```python
from build123d import *

# Parameters (mm, degrees)
STOCK_LED_START                   = -2.54
STOCK_LED_LIGHT_HOUSING_1_DEPTH   = 2.54
STOCK_LED_LIGHT_HOUSING_1_2_DEPTH = 13.97
SKETCH3_W                         = 2.54
SKETCH3_H                         = 17.78
PIECE_UNDER_BATTERY_PLUG_DEPTH    = 7.62
CUT_OUT_FOR_PLUG_REACH            = 94.065
SKETCH4_R                         = 5.157413323
HOLES_FOR_SCREWS_D                = 3.2639
SKETCH7_W                         = 25.4
SKETCH7_H                         = 12.726484406
SKETCH7_W_2                       = 12.813224924
SKETCH7_H_2                       = 12.784135739
NAILS_GO_HERE_DEPTH               = 3.81
NAIL_HOLES_D                      = 3.2639
FILLET1_R                         = 2.54


# Read off the part's stored shape, not the designer's step: Stock-LED Light housing-1
with BuildPart() as part:
    # Stock-LED Light housing-1 outline → Stock-LED Light housing-1 (new body)
    with BuildSketch(Plane(origin=(0, 0, 0), x_dir=(1, 0, 0), z_dir=(0, 1, 0)).offset(STOCK_LED_START)):
        Polygon((71.203772107, -22.802348667), (71.203772107, 38.157651333), (-11.408866572, 38.157651333), (-11.408866572, 0.057651333), (-42.066153873, 0.057651333), (-42.066153873, -22.802348667), align=None)
    extrude(amount=STOCK_LED_LIGHT_HOUSING_1_DEPTH)

    # Stock-LED Light housing-1 2 outline → Stock-LED Light housing-1 2 (add)
    with BuildSketch(Plane(origin=(0, 0, 0), x_dir=(1, 0, 0), z_dir=(0, 1, 0))):
        Polygon((71.203772107, -22.802348667), (71.203772107, 38.157651333), (-11.408866572, 38.157651333), (-11.408866572, 0.057651333), (-42.066153873, 0.057651333), (-42.066153873, -22.802348667), align=None)
        Polygon((-39.526153873, -20.262348667), (-39.526153873, -2.482348667), (-8.868866572, -2.482348667), (-8.868866572, 35.617651333), (68.663772107, 35.617651333), (68.663772107, -20.262348667), align=None, mode=Mode.SUBTRACT)
    extrude(amount=STOCK_LED_LIGHT_HOUSING_1_2_DEPTH)

    # Sketch3 → Piece under battery plug (add)
    with BuildSketch(Plane(origin=(0, 0, 0), x_dir=(1, 0, 0), z_dir=(0, 1, 0))):
        with Locations((-10.138866572, -11.372348667)):
            Rectangle(SKETCH3_W, SKETCH3_H)
    extrude(amount=PIECE_UNDER_BATTERY_PLUG_DEPTH)

    # Sketch4 → Cut out for plug (cut, up to next)
    with BuildSketch(Plane(origin=(-11.408866572, 0, 0), x_dir=(0, 0, -1), z_dir=(1, 0, 0)), mode=Mode.PRIVATE) as cut_out_for_plug_sk1:
        with Locations((-11.372348667, 7.62)):
            Circle(SKETCH4_R)
    cut_out_for_plug_tool1 = extrude(cut_out_for_plug_sk1.sketch, amount=CUT_OUT_FOR_PLUG_REACH, mode=Mode.PRIVATE) & part.part
    add(cut_out_for_plug_tool1.solids().sort_by_distance((-11.408867, 7.62, 11.372349))[0], mode=Mode.SUBTRACT)

    # holes for screws (through all)
    with Locations(Plane(origin=(0, 0, 0), x_dir=(1, 0, 0), z_dir=(0, 1, 0))):
        with Locations((14.053772107, 31.922137324), (12.783772107, -16.337862676), (64.853772107, -11.257862676), (64.853772107, 16.682137324)):
            Hole(HOLES_FOR_SCREWS_D / 2)

    # Sketch7 → Nails go here (add)
    with BuildSketch(Plane(origin=(0, 13.97, 0), x_dir=(1, 0, 0), z_dir=(0, 1, 0))):
        with Locations((-24.108866572, 6.420893536)):
            Rectangle(SKETCH7_W, SKETCH7_H)
        with Locations((77.610384569, 6.39206787)):
            Rectangle(SKETCH7_W_2, SKETCH7_H_2)
    extrude(amount=-NAILS_GO_HERE_DEPTH)

    # Nail holes (through all)
    with Locations(Plane(origin=(0, 10.16, 0), x_dir=(-1, 0, 0), z_dir=(0, -1, 0))):
        with Locations((30.430786564, 6.434135739), (-77.666997031, 6.434135739)):
            Hole(NAIL_HOLES_D / 2)

    # Fillet1
    fillet1_edges = [part.edges().sort_by_distance(p)[0] for p in [
        (71.203772107, 5.715, -38.157651333),
        (71.203772107, 5.715, 22.802348667),
        (-36.808866572, 10.16, -6.420893536),
        (-24.108866572, 10.16, -12.784135739),
        (-36.808866572, 12.065, -12.784135739),
        (77.610384569, 10.16, -12.784135739),
        (84.016997031, 10.16, -6.392067869),
        (84.016997031, 12.065, -12.784135739),
        (77.610384569, 10.16, 0),
        (84.016997031, 12.065, 0),
        (-26.737510222, -2.54, -0.057651333),
        (14.568809117, -2.54, 22.802348667),
        (29.897452767, -2.54, -38.157651333),
        (-42.066153873, 5.715, 22.802348667),
        (-42.066153873, 5.715, -0.057651333),
        (-42.066153873, -2.54, 11.372348667),
        (71.203772107, -2.54, -7.677651333),
        (-11.408866572, 5.715, -38.157651333),
        (-11.408866572, -2.54, -19.107651333),
    ]]
    fillet(fillet1_edges, radius=FILLET1_R)


solid = part.part
```
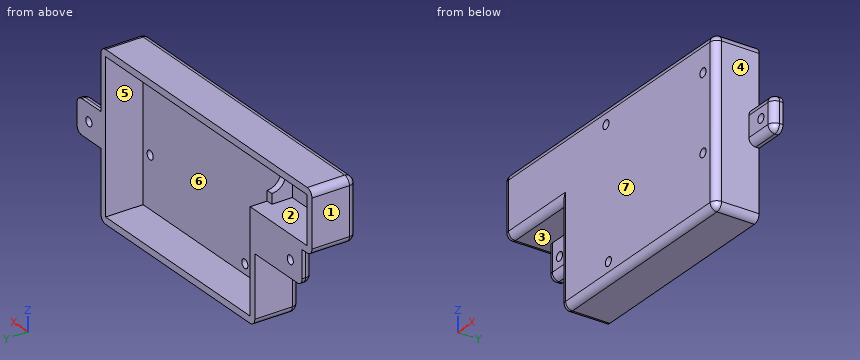
Check sheet for the modelled part. Datum: model origin and axes. Units: mm. Face numbers are marked on the shaded views. A direction names the side the tool comes from. Give positions to 0.01 mm unless a question says otherwise; leave off trailing zeros. Order: outer loops, then holes, each group sorted by start corner. A loop starts at its lowest first (then second) coordinate and runs counter-clockwise, first axis right, second up. Notation, with made-up numbers: M 54.25,-7 L 100.25,-7 A16 cw 100.25,20 Z; hole C -37,55.5 d6. An arc over 180 degrees is marked long. Answer in a Markdown table with one row per item. Add a question column.
Q1. Release check for a two-part mould opening along X. For the marked faces 4, 5, 6 and 7 record: released by +X, released by -X, zero draft, split by the parting line, or undercut.
Q2. Sectioned sample at D-D, the plane x = 59.5. Record the boundary of the cut face in (y, z).
Q3. Access from +Z, -Z, +X, -X, +Y, -Y to the whole of each face (thin tool, end or side, straight path). Record for the marked faces 1, 2 and 3.
Q4. Sectioned sample at B-B, the plane z = 5. Record the boundary of the cut face in (x, y), and give its area (3 significant figures).
Q5. Sectioned sample at A-A, the plane y = 8.75. Record the boundary of the cut face in (x, z), and give its area (3 significant figures).
Q6. Gauge pin test, flat ends, axial feed: pin 1 Ø4 at (y, z) = (8.5, -1.5) entering from +X; pin 2 Ø5 at (y, z) = (0, -27.5) entering from +X; pin 3 Ø1 at (x, y) = (76.5, 13.5) entering from +Z. Record the tip position at first contact, or that the pin passes through.
Q7. Thickness scan on L1, parallel to X at y = 6.25, z = 4; L2, parallel to X at y = 7, z = 11; L3, parallel to Z at x = 32.5, y = 6.5. Record the ranges inside material, lowest first.
Q8. Sectioned sample at C-C, the plane x = -25. Record the boundary of the cut face in (y, z), and give its area (3 significant figures).
Verdict:
| question | item | result |
|---|---|---|
| 1 | face 4 | released by +X |
| 1 | face 5 | undercut |
| 1 | face 6 | undercut |
| 1 | face 7 | zero draft |
| 2 | outline | M -2.54,-35.62 A2.54 ccw 0,-38.16 L 13.97,-38.16 L 13.97,-35.62 L 0,-35.62 L 0,20.26 L 13.97,20.26 L 13.97,22.8 L 0,22.8 A2.54 ccw -2.54,20.26 Z |
| 3 | face 1 | +Z, -Z, -X, +Y, -Y |
| 3 | face 2 | +Y |
| 3 | face 3 | -Z, -X, -Y |
| 4 | outline | M -42.07,0 A2.54 ccw -39.53,-2.54 L 68.66,-2.54 A2.54 ccw 71.2,0 L 71.2,13.97 L 68.66,13.97 L 68.66,0 L -8.87,0 L -8.87,7.62 L -11.41,7.62 L -11.41,0 L -39.53,0 L -39.53,13.97 L -42.07,13.97 Z |
| 4 | area | 375 mm² |
| 5 | outline | M -42.07,2.48 A2.54 ccw -39.53,-0.06 L -11.41,-0.06 L -11.41,-35.62 A2.54 ccw -8.87,-38.16 L 68.66,-38.16 A2.54 ccw 71.2,-35.62 L 71.2,20.26 A2.54 ccw 68.66,22.8 L -39.53,22.8 A2.54 ccw -42.07,20.26 Z; hole M -39.53,2.48 L -8.87,2.48 L -8.87,-35.62 L 68.66,-35.62 L 68.66,20.26 L -39.53,20.26 Z |
| 5 | area | 852 mm² |
| 6 | pin 1 | x = 82.5 |
| 6 | pin 2 | x = 71.2 |
| 6 | pin 3 | z = 0 |
| 7 | L1 | -42.07 to -39.53, -11.41 to -8.87, 68.66 to 71.2 |
| 7 | L2 | -42.07 to -39.53, 68.66 to 71.2 |
| 7 | L3 | -38.16 to -35.62, 20.26 to 22.8 |
| 8 | outline | M -2.54,2.48 A2.54 ccw 0,-0.06 L 10.16,-0.06 L 10.16,-10.24 A2.54 ccw 12.7,-12.78 L 13.97,-12.78 L 13.97,2.48 L 0,2.48 L 0,20.26 L 13.97,20.26 L 13.97,22.8 L 0,22.8 A2.54 ccw -2.54,20.26 Z |
| 8 | area | 173 mm² |
